Source: three-view drawing plus pictorial views. Frame: mm from the lowest corner of the part. A direction names the side the tool comes from. Give positions to 0.01 mm unless a question says otherwise; leave off trailing zeros. Loops run counter-clockwise (first coordinate to the right, second up) from the corner with the lowest first, then second, coordinate; pieces in that order, holes last.
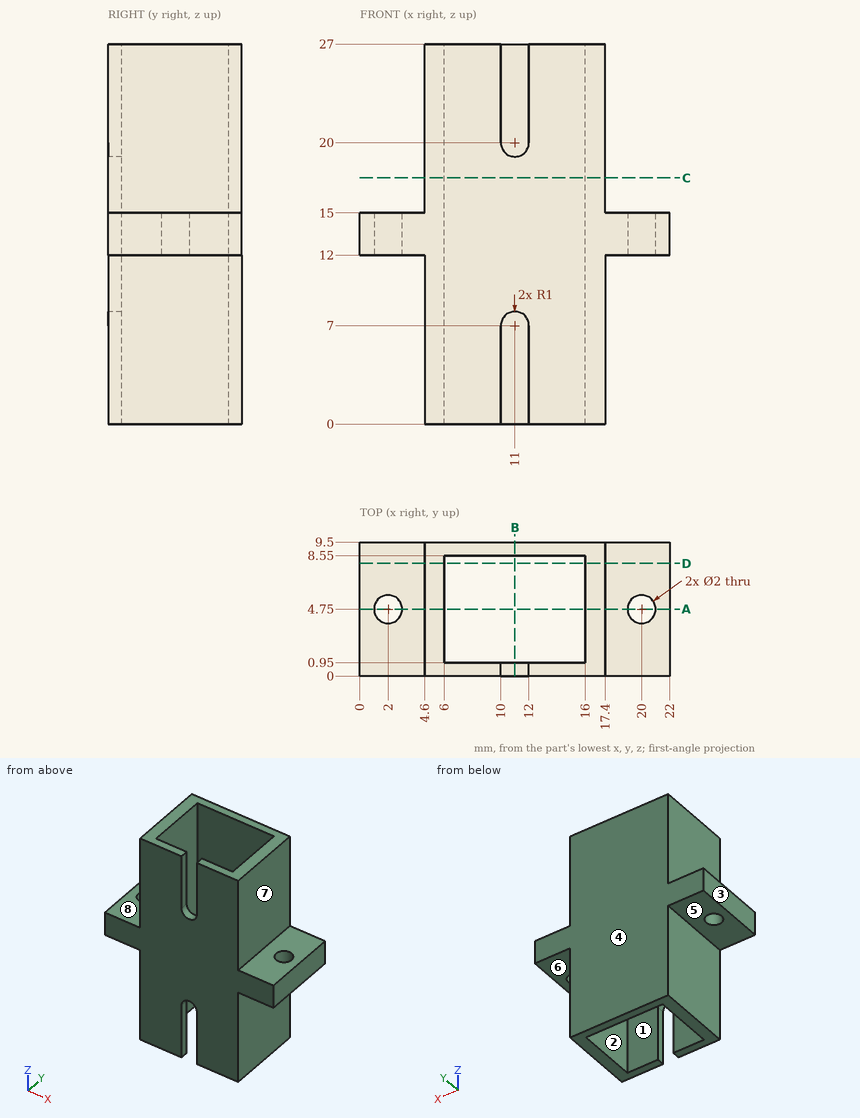
(1) Mould query, pull axis Y, two halves, no side actions, for the marked faces 1, 2, 3 and 4. Classes: +Y half, -Y half, draft (parallel to the pull), parting line (faces both ways), or undercut.
Values follow:
face 1: undercut
face 2: undercut
face 3: draft
face 4: +Y half
(2) Ray query, probe 1 along Y at (x, z) = (20, 12.95); probe 2 along Y at (x, z) = (12, 11); probe 3 along X at (y, z) = (5.75, 7). Return the intervals inside material, ascending.
Values follow:
probe 1: y = 0 to 3.75, 5.75 to 9.5
probe 2: y = 0 to 0.95, 8.55 to 9.5
probe 3: x = 4.6 to 6, 16 to 17.4
(3) Reachability of the marked faces 5, 6, 7 and 8 from +Z, -Z, +X, -X, +Y, -Y: full face, straight path, thin tool, end or side. Return the list, or none.
Values follow:
face 5: -Z, -X, +Y, -Y
face 6: -Z, +X, +Y, -Y
face 7: +Z, +X, +Y, -Y
face 8: +Z, -X, +Y, -Y
(4) Cut plane C-C (z = 17.5). Return the cut outline in (x, y), and give its area (3 significant figures).
Values follow:
outline: (4.6, 0) - (17.4, 0) - (17.4, 9.5) - (4.6, 9.5) - close; hole (6, 0.95) - (16, 0.95) - (16, 8.55) - (6, 8.55) - close
area: 45.6 mm2
(5) Cut plane D-D (y = 8). Return the cut outline in (x, z), and give its area (3 significant figures).
Values follow:
outline: (0, 12) - (4.6, 12) - (4.6, 0) - (6, 0) - (6, 27) - (4.6, 27) - (4.6, 15) - (0, 15) - close; (16, 0) - (17.4, 0) - (17.4, 12) - (22, 12) - (22, 15) - (17.4, 15) - (17.4, 27) - (16, 27) - close
area: 103 mm2
(6) Pin query (flat end, axial travel): pin 1 Ø3 at (x, y) = (3.5, 6.5) entering from +Z; pin 2 Ø1.4 at (x, y) = (3, 6.5) entering from +Z; pin 3 Ø0.5 at (y, z) = (0.5, 22.5) entering from +X; pin 4 Ø2.5 at (x, y) = (20, 4.75) entering from -Z. Return the tip coordinate at first contact, or that it passes through.
Values follow:
pin 1: stops at z = 27
pin 2: stops at z = 15
pin 3: stops at x = 17.4
pin 4: stops at z = 12
(7) Cut plane A-A (y = 4.75). Return the cut outline in (x, z), and give its area (3 significant figures).
Values follow:
outline: (0, 12) - (1, 12) - (1, 15) - (0, 15) - close; (3, 12) - (4.6, 12) - (4.6, 0) - (6, 0) - (6, 27) - (4.6, 27) - (4.6, 15) - (3, 15) - close; (16, 0) - (17.4, 0) - (17.4, 12) - (19, 12) - (19, 15) - (17.4, 15) - (17.4, 27) - (16, 27) - close; (21, 12) - (22, 12) - (22, 15) - (21, 15) - close
area: 91.2 mm2
(8) Cut plane B-B (x = 11). Return the cut outline in (y, z), and give its area (3 significant figures).
Values follow:
outline: (0, 8) - (0.95, 8) - (0.95, 19) - (0, 19) - close; (8.55, 0) - (9.5, 0) - (9.5, 27) - (8.55, 27) - close
area: 36.1 mm2
